Design review of the part shown in the three views and the two pictorial views. Dimensions are in mm from the part's minimum x, y and z. Coordinates: 2 decimals unless noted, no trailing zeros. Loops run counter-clockwise (first coordinate to the right, second up) from the corner with the lowest first, then second, coordinate; pieces in that order, holes last. Notation, with made-up numbers: (-10.5, -5.75) -> (-2.5, -5.75) arc R4 ccw to (-2.5, -1.75) -> close; hole circle Ø5 at (7.5, 36). An arc over 180 degrees is marked (long way). Use CSV: the item, a comma, the result in double quotes.
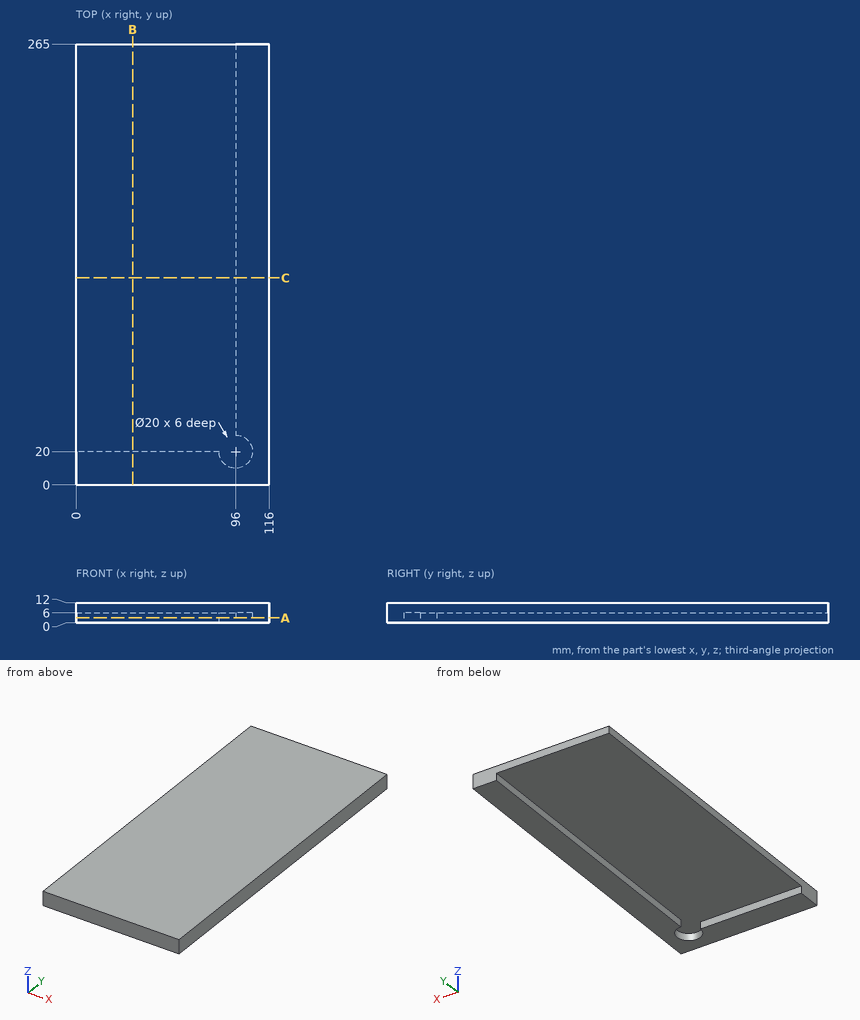
Item 1: Add section A-A (z = 3). Give the boundary of the cut face in (x, y).
Checked values:
outline,"(0, 0) -> (116, 0) -> (116, 265) -> (96, 265) -> (96, 30) arc R10 cw (long way) to (86, 20) -> (0, 20) -> close"
Item 2: Add section B-B (x = 34). Give the boundary of the cut face in (y, z), then the cut area to 3 significant figures.
Checked values:
outline,"(0, 0) -> (20, 0) -> (20, 6) -> (265, 6) -> (265, 12) -> (0, 12) -> close"
area,"1,710 mm^2"
Item 3: Add section C-C (y = 124.5). Give the boundary of the cut face in (x, z), then the cut area to 3 significant figures.
Checked values:
outline,"(0, 6) -> (96, 6) -> (96, 0) -> (116, 0) -> (116, 12) -> (0, 12) -> close"
area,"816 mm^2"
Item 4: Clearance check with flat-ended pins moving along their axes: pin 1 (5 mm diameter, centred on x = 89, y = 176, fed in from -Z); pin 2 (5 mm diameter, centred on x = 26, z = 2, fed in from +Y). State where each tip first meets the part, or that it passes through.
Checked values:
pin 1,"z = 6"
pin 2,"y = 20"
Item 5: To check wall thickness, follow line 1 along Z through (x, y) = (19, 232); line 2 along X through (y, z) = (77, 4.75); line 3 along Y through (x, z) = (80, 2.75). State the ranges of each line that lie inside material, in increasing order.
Checked values:
line 1,"6 to 12"
line 2,"96 to 116"
line 3,"0 to 20"
